For this review, take the finished solid that the model builds, in its own axes (mm). Face numbers are marked on the shaded views. Give positions to 0.01 mm unless a question says otherwise; leave off trailing zeros. Loops run counter-clockwise (first coordinate to the right, second up) from the corner with the lowest first, then second, coordinate; pieces in that order, holes last. Notation, with made-up numbers: (66.5, 6) - (92.5, 6) arc R29 cw to (92.5, 33) - close; hole circle Ø9 at (12, -18.5). An arc over 180 degrees is marked (long way). Put each result on its own line as item: value.
from build123d import *

# Parameters (mm, degrees)
ESTRUSIONE_ESTRUSIONE1_DEPTH = 140
ESTRUSIONE_ESTRUSIONE2_START = -5
ESTRUSIONE_ESTRUSIONE2_DEPTH = 5
ESTRUSIONE_ESTRUSIONE3_DEPTH = 5
SCHIZZO4_W                   = 65
SCHIZZO4_H                   = 65
TAGLIO_ESTRUSIONE1_DEPTH     = 190.601391721
SCHIZZO6_W                   = 80
SCHIZZO6_H                   = 80
SCHIZZO6_W_2                 = 72
SCHIZZO6_H_2                 = 72
ESTRUSIONE_ESTRUSIONE5_DEPTH = 10.61
SCHIZZO8_W                   = 10
SCHIZZO8_H                   = 6
ESTRUSIONE_ESTRUSIONE6_DEPTH = 8
SCHIZZO9_R                   = 1.5
TAGLIO_ESTRUSIONE2_DEPTH     = 5
TAGLIO_ESTRUSIONE3_DEPTH     = 314.596874984
RACCORDO1_R                  = 10


with BuildPart() as part:
    # Schizzo1 → Estrusione-Estrusione1 (new body)
    with BuildSketch(Plane.XY):
        with BuildLine():
            Line((121.383689184, -221.979728804), (115, -221.979728804))
            ThreePointArc((115, -221.979728804), (0, -250), (-115, -221.979728804))
            Line((-115, -221.979728804), (-121.383689184, -221.979728804))
            ThreePointArc((-121.383689184, -221.979728804), (0, -253), (121.383689184, -221.979728804))
        make_face()
    extrude(amount=ESTRUSIONE_ESTRUSIONE1_DEPTH)

    # Schizzo2 → Estrusione-Estrusione2 (add)
    with BuildSketch(Plane.XY.offset(140).offset(ESTRUSIONE_ESTRUSIONE2_START)):
        with BuildLine():
            Line((-121.383689184, -218.554341069), (-121.383689184, -221.979728804))
            Line((-121.383689184, -221.979728804), (-115, -221.979728804))
            ThreePointArc((-115, -221.979728804), (-118.204253089, -220.290159906), (-121.383689184, -218.554341069))
        make_face()
        with BuildLine():
            Line((-121.383689184, -212.816822643), (-121.383689184, -218.554341069))
            ThreePointArc((-121.383689184, -218.554341069), (-118.204253089, -220.290159906), (-115, -221.979728804))
            ThreePointArc((-115, -221.979728804), (0, -250), (115, -221.979728804))
            ThreePointArc((115, -221.979728804), (118.204253089, -220.290159906), (121.383689184, -218.554341069))
            Line((121.383689184, -218.554341069), (121.383689184, -212.816822643))
            ThreePointArc((121.383689184, -212.816822643), (0, -245), (-121.383689184, -212.816822643))
        make_face()
        with BuildLine():
            Line((115, -221.979728804), (121.383689184, -221.979728804))
            Line((121.383689184, -221.979728804), (121.383689184, -218.554341069))
            ThreePointArc((121.383689184, -218.554341069), (118.204253089, -220.290159906), (115, -221.979728804))
        make_face()
    extrude(amount=ESTRUSIONE_ESTRUSIONE2_DEPTH)

    # Schizzo3 → Estrusione-Estrusione3 (add)
    with BuildSketch(Plane(origin=(0, 0, 0), x_dir=(-1, 0, 0), z_dir=(0, 0, -1))):
        with BuildLine():
            Line((-121.383689184, -212.816822643), (-121.383689184, -218.554341069))
            ThreePointArc((-121.383689184, -218.554341069), (-118.204253089, -220.290159906), (-115, -221.979728804))
            ThreePointArc((-115, -221.979728804), (0, -250), (115, -221.979728804))
            ThreePointArc((115, -221.979728804), (118.204253089, -220.290159906), (121.383689184, -218.554341069))
            Line((121.383689184, -218.554341069), (121.383689184, -212.816822643))
            ThreePointArc((121.383689184, -212.816822643), (0, -245), (-121.383689184, -212.816822643))
        make_face()
        with BuildLine():
            Line((115, -221.979728804), (121.383689184, -221.979728804))
            Line((121.383689184, -221.979728804), (121.383689184, -218.554341069))
            ThreePointArc((121.383689184, -218.554341069), (118.204253089, -220.290159906), (115, -221.979728804))
        make_face()
        with BuildLine():
            Line((-121.383689184, -218.554341069), (-121.383689184, -221.979728804))
            Line((-121.383689184, -221.979728804), (-115, -221.979728804))
            ThreePointArc((-115, -221.979728804), (-118.204253089, -220.290159906), (-121.383689184, -218.554341069))
        make_face()
    extrude(amount=-ESTRUSIONE_ESTRUSIONE3_DEPTH)

    # Schizzo4 → Taglio-Estrusione1 (cut, through all)
    with BuildSketch(Plane(origin=(0, -253, 0), x_dir=(-1, 0, 0), z_dir=(0, -1, 0))):
        with Locations((0, -70)):
            Rectangle(SCHIZZO4_W, SCHIZZO4_H)
    extrude(amount=-TAGLIO_ESTRUSIONE1_DEPTH, mode=Mode.SUBTRACT)

    # Schizzo6 → Estrusione-Estrusione5 (add)
    with BuildSketch(Plane(origin=(0, -253, 0), x_dir=(-1, 0, 0), z_dir=(0, -1, 0))):
        with Locations((0, -70)):
            Rectangle(SCHIZZO6_W, SCHIZZO6_H)
        with Locations((0, -70)):
            Rectangle(SCHIZZO6_W_2, SCHIZZO6_H_2, mode=Mode.SUBTRACT)
    extrude(amount=-ESTRUSIONE_ESTRUSIONE5_DEPTH)

    # Schizzo8 → Estrusione-Estrusione6 (add)
    with BuildSketch(Plane(origin=(0, -242.39, 0), x_dir=(1, 0, 0), z_dir=(0, 1, 0))):
        with Locations((0, -27)):
            Rectangle(SCHIZZO8_W, SCHIZZO8_H)
        with Locations((0, -113)):
            Rectangle(SCHIZZO8_W, SCHIZZO8_H)
    extrude(amount=-ESTRUSIONE_ESTRUSIONE6_DEPTH)

    # Schizzo9 → Taglio-Estrusione2 (cut)
    with BuildSketch(Plane(origin=(0, -242.39, 0), x_dir=(1, 0, 0), z_dir=(0, 1, 0))):
        with Locations(Location((0, -29, 0), (0, 0, 270))):
            Circle(SCHIZZO9_R)
        with Locations(Location((0, -111, 0), (0, 0, 270))):
            Circle(SCHIZZO9_R)
    extrude(amount=-TAGLIO_ESTRUSIONE2_DEPTH, mode=Mode.SUBTRACT)

    # Schizzo10 → Taglio-Estrusione3 (cut, through all)
    with BuildSketch(Plane(origin=(0, 0, 0), x_dir=(-1, 0, 0), z_dir=(0, 0, -1))):
        with BuildLine():
            Line((-121.383689184, -295.114305534), (125.369855002, -295.114305534))
            Line((125.369855002, -295.114305534), (121.383689184, -221.979728804))
            ThreePointArc((121.383689184, -221.979728804), (0, -253), (-121.383689184, -221.979728804))
            Line((-121.383689184, -221.979728804), (-121.383689184, -295.114305534))
        make_face()
    extrude(amount=-TAGLIO_ESTRUSIONE3_DEPTH, mode=Mode.SUBTRACT)

    # Raccordo1
    # the kernel refuses this fillet: 10 mm, written as the material it adds along each edge
    with BuildSketch(Plane(origin=(5, -249.949994999, 55.515759856), x_dir=(0.999183410527211, 0.04040435777500708, 0), z_dir=(0, 0, -1))) as raccordo1_piece_1_section:
        with BuildLine():
            CenterArc((10.002177863, -9.99791641), RACCORDO1_R, 88.830362483, 77.02269885)
            Line((0.305456743, -7.553821587), (0, 0))
            ThreePointArc((0, 0), (5.103151971, 0.052089747), (10.206303942, 0))
        make_face()
    raccordo1_piece_1 = extrude(amount=31.515759856, mode=Mode.PRIVATE)
    raccordo1_piece_1 = split(raccordo1_piece_1, bisect_by=Plane(origin=(10.036552928, -248.481695624, 34), z_dir=(0, 0, -1)), keep=Keep.TOP, mode=Mode.PRIVATE)
    add(raccordo1_piece_1)
    with BuildSketch(Plane(origin=(40, -246.779253585, 110), x_dir=(0.9840071168859134, 0.17812914954569523, 0), z_dir=(0, 0, -1))) as raccordo1_piece_2:
        with BuildLine():
            CenterArc((9.012656027, -9.998308312), RACCORDO1_R, 88.946089238, 56.448243915)
            Line((0.781854008, -4.319056766), (0, 0))
            ThreePointArc((0, 0), (4.598293891, 0.042292191), (9.196587782, 0))
        make_face()
    extrude(amount=80)
    with BuildSketch(Plane(origin=(5, -249.949994999, 116), x_dir=(0.9991834105272109, 0.04040435777500963, 0), z_dir=(0, 0, -1))) as raccordo1_piece_3_section:
        with BuildLine():
            CenterArc((10.002177863, -9.99791641), RACCORDO1_R, 88.830362483, 77.02269885)
            Line((0.305456743, -7.553821587), (0, 0))
            ThreePointArc((0, 0), (5.103151971, 0.052089747), (10.206303942, 0))
        make_face()
    raccordo1_piece_3 = extrude(amount=31.515759856, mode=Mode.PRIVATE)
    raccordo1_piece_3 = split(raccordo1_piece_3, bisect_by=Plane(origin=(10.036552928, -248.481695624, 106), z_dir=(0, 0, 1)), keep=Keep.TOP, mode=Mode.PRIVATE)
    add(raccordo1_piece_3)
    with BuildSketch(Plane(origin=(-5, -249.949994999, 116), x_dir=(-0.9991834105272109, 0.04040435777501259, 0), z_dir=(0, 0, -1))) as raccordo1_piece_4_section:
        with BuildLine():
            CenterArc((10.002177863, 9.99791641), RACCORDO1_R, 194.146938667, 77.02269885)
            Line((0.305456743, 7.553821587), (0, 0))
            ThreePointArc((0, 0), (5.103151971, -0.052089747), (10.206303942, 0))
        make_face()
    raccordo1_piece_4 = extrude(amount=31.515759856, mode=Mode.PRIVATE)
    raccordo1_piece_4 = split(raccordo1_piece_4, bisect_by=Plane(origin=(-10.036552928, -248.481695624, 106), z_dir=(0, 0, 1)), keep=Keep.TOP, mode=Mode.PRIVATE)
    add(raccordo1_piece_4)
    with BuildSketch(Plane(origin=(-40, -246.779253585, 110), x_dir=(-0.9840071168859144, 0.17812914954568923, 0), z_dir=(0, 0, -1))) as raccordo1_piece_5:
        with BuildLine():
            CenterArc((9.012656027, 9.998308312), RACCORDO1_R, 214.605666847, 56.448243915)
            Line((0.781854008, 4.319056766), (0, 0))
            ThreePointArc((0, 0), (4.598293891, -0.042292191), (9.196587782, 0))
        make_face()
    extrude(amount=80)
    with BuildSketch(Plane(origin=(-5, -249.949994999, 55.515759856), x_dir=(-0.9991834105272107, 0.040404357775012466, 0), z_dir=(0, 0, -1))) as raccordo1_piece_6_section:
        with BuildLine():
            CenterArc((10.002177863, 9.99791641), RACCORDO1_R, 194.146938667, 77.02269885)
            Line((0.305456743, 7.553821587), (0, 0))
            ThreePointArc((0, 0), (5.103151971, -0.052089747), (10.206303942, 0))
        make_face()
    raccordo1_piece_6 = extrude(amount=31.515759856, mode=Mode.PRIVATE)
    raccordo1_piece_6 = split(raccordo1_piece_6, bisect_by=Plane(origin=(-10.036552928, -248.481695624, 34), z_dir=(0, 0, -1)), keep=Keep.TOP, mode=Mode.PRIVATE)
    add(raccordo1_piece_6)


solid = part.part
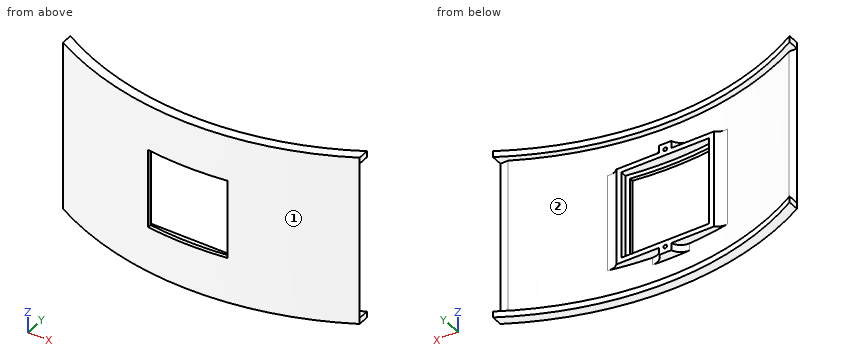
1) Take a section at C-C on z = 80.5. State the section outline as (x, y) points, and give its area (3 significant figures).
Geometry check:
outline: (-121.38, -221.98) arc R253 ccw to (-32.5, -250.9) - (-32.5, -247.88) arc R250 cw to (-36, -247.39) - (-36, -242.39) - (-40, -242.39) arc R10 cw to (-49.05, -245.14) arc R250 cw to (-115, -221.98) - close; (32.5, -250.9) arc R253 ccw to (121.38, -221.98) - (115, -221.98) arc R250 cw to (49.05, -245.14) arc R10 cw to (40, -242.39) - (36, -242.39) - (36, -247.39) arc R250 cw to (32.5, -247.88) - close
area: 606 mm²
2) Take a section at A-A on y = -216. State the section outline as (x, z) points.
Geometry check:
outline: (-121.38, 0) - (-115.62, 0) - (-115.62, 5) - (-121.38, 5) - close; (-121.38, 135) - (-115.62, 135) - (-115.62, 140) - (-121.38, 140) - close; (115.62, 0) - (121.38, 0) - (121.38, 5) - (115.62, 5) - close; (115.62, 135) - (121.38, 135) - (121.38, 140) - (115.62, 140) - close
3) Wall thickness on line 1 (Z direction, x = 19, y = -248); line 2 (Z direction, x = -62.5, y = -241.5); line 3 (X direction, y = -225, z = 94): over which ranges is each line inside the solid? List them lowest first.
Geometry check:
line 1: z = 0 to 5, 30 to 34, 106 to 110, 135 to 140
line 2: z = 0 to 5, 135 to 140
line 3: x = -115.69 to -108.97, 108.97 to 115.69
4) Take a section at D-D on x = 67. State the section outline as (y, z) points, and give its area (3 significant figures).
Geometry check:
outline: (-243.97, 0) - (-235.66, 0) - (-235.66, 5) - (-240.85, 5) - (-240.85, 135) - (-235.66, 135) - (-235.66, 140) - (-243.97, 140) - close
area: 488 mm²
5) Draft analysis for pull direction X (two halves, no side actions). For the marked faces 1 and 2, state which applies: pulls with the +X half, pulls with the -X half, needs draft (parallel to the pull), parting line crosses it, or undercut.
Geometry check:
face 1: parting line crosses it
face 2: undercut
6) Insertion check: pin 1 Ø3.5 at (x, y) = (-19.5, -246.5) entering from -Z; pin 2 Ø1.5 at (x, z) = (0, 29.5) entering from +Y; pin 3 Ø6 at (y, z) = (-233, 56) entering from -X; pin 4 Ø7 at (x, z) = (-117.5, 92.5) entering from +Y. Each pin has a flat end and moves straight along its axis. Give the tip position at first contact, or say it passes through.
Geometry check:
pin 1: stops at z = 0
pin 2: stops at y = -247.39
pin 3: stops at x = -105.4
pin 4: stops at y = -221.98
